Can you work these out from the model? Positions are in its coordinate system, mm. A direction names the side the tool comes from. Give positions to 0.01 mm unless a question says otherwise; leave off trailing zeros. Order: outer loops, then holes, each group sorted by start corner. A loop starts at its lowest first (then second) coordinate and runs counter-clockwise, first axis right, second up. Notation, with made-up numbers: M 15.5,-22.5 L 20.5,-22.5 A19 cw 20.5,9.5 Z; hole C 62,-14 d11. An arc over 180 degrees is marked long. One line per question, with ' | ' between items. Start each with the question number.
1) I'm going to push flat-ended pins straight in: pin 1 Ø10 at (y, z) = (-773, 4.5) entering from +X; pin 2 Ø5 at (x, z) = (-20.5, 11) entering from -Y; pin 3 Ø5 at (y, z) = (-780, 2) entering from -X. Where does each tip first touch, or does it pass through?
2) If we section it at C-C, the plane y = -778: Please give me the cut outline in (x, z) (3 decimals).
3) If we section it at B-B, the plane x = -28: Please give me the cut outline in (y, z) (3 decimals), plus the area to 3 significant figures.
4) If we section it at A-A, the plane z = 0: Please give me the cut outline in (x, y).
5) For faces 4 (the flat face through (-16, -775, -9.525)), 5 (the cylindrical face through (-7.9, -759.1, -12.1)), which set-ups out of +Z, -Z, +X, -X, +Y, -Y let a thin tool reach every point of the face, with its end or its side?
6) If we section it at D-D, the plane y = -766.5: Please give me the cut outline in (x, z) (3 decimals).
7) Please list where these lines run through material, in increasing order: line 1 along Z through (x, y) = (-9, -783) (3 decimals); line 2 along X through (y, z) = (-762.5, -2.5); line 3 along Y through (x, z) = (-27.5, -10.5). Write a range as [from, to].
8) Thinking about a two-plate mould opening in Y: for faces 1 (the flat face through (-3, -759.052, 0)), 2 (the cylindrical face through (-23.005, -779.083, 12.101)), 3 (the flat face through (-34.362, -776, 12)), which applies, +Y half, -Y half, draft (parallel to the pull), parting line (faces both ways), or undercut?
```python
from build123d import *

# Parameters (mm, degrees)
BOSS_EXTRUDE1_DEPTH = 33.02
CUT_EXTRUDE1_REACH  = 794.952
SKETCH2_R           = 3.175
SKETCH3_R           = 3.96875
CUT_EXTRUDE2_DEPTH  = 794.354962335
FILLET1_R           = 3.175


with BuildPart() as part:
    # Sketch1 → Boss-Extrude1 (new body)
    with BuildSketch(Plane(origin=(0, -759.052062329, 0), x_dir=(-1, 0, 0), z_dir=(0, -1, 0))):
        Polygon((0, 14.605), (0, -14.605), (34.361609966, -14.605), (34.361609966, -9.525), (5.08, -9.525), (5.08, 9.525), (34.361609966, 9.525), (34.361609966, 14.605), align=None)
    extrude(amount=BOSS_EXTRUDE1_DEPTH)

    # Sketch2 → Cut-Extrude1 (cut, up to next)
    with BuildSketch(Plane(origin=(0, 0, 0), x_dir=(0, 0, -1), z_dir=(1, 0, 0)), mode=Mode.PRIVATE) as cut_extrude1_sk1:
        with Locations(Location((0, -784.452062329, 0), (0, 0, 90))):
            Circle(SKETCH2_R)
    cut_extrude1_tool1 = extrude(cut_extrude1_sk1.sketch, amount=-CUT_EXTRUDE1_REACH, mode=Mode.PRIVATE) & part.part
    # Sketch2 → Cut-Extrude1 (cut, up to next)
    with BuildSketch(Plane(origin=(0, 0, 0), x_dir=(0, 0, -1), z_dir=(1, 0, 0)), mode=Mode.PRIVATE) as cut_extrude1_sk2:
        with Locations(Location((0, -766.672062329, 0), (0, 0, 90))):
            Circle(SKETCH2_R)
    cut_extrude1_tool2 = extrude(cut_extrude1_sk2.sketch, amount=-CUT_EXTRUDE1_REACH, mode=Mode.PRIVATE) & part.part
    add(cut_extrude1_tool1.solids().sort_by_distance((0, -784.452062, 0))[0], mode=Mode.SUBTRACT)
    add(cut_extrude1_tool2.solids().sort_by_distance((0, -766.672062, 0))[0], mode=Mode.SUBTRACT)

    # Sketch3 → Cut-Extrude2 (cut, through all)
    with BuildSketch(Plane.XY.offset(14.605)):
        with Locations((-24.836609966, -775.562062329)):
            Circle(SKETCH3_R)
        Polygon((-7.9375, -759.052062329), (-34.361609966, -769.212062329), (-34.361609966, -759.052062329), align=None)
        Polygon((-34.361609966, -792.072062329), (-34.361609966, -781.912062329), (-7.9375, -792.072062329), align=None)
    extrude(amount=-CUT_EXTRUDE2_DEPTH, mode=Mode.SUBTRACT)

    # Fillet1
    fillet1_edges = [part.edges().sort_by_distance(p)[0] for p in [
        (-7.9375, -759.052062329, 12.065),
        (-7.9375, -792.072062329, 12.065),
        (-34.361609966, -781.912062329, 12.065),
        (-7.9375, -792.072062329, -12.065),
        (-34.361609966, -781.912062329, -12.065),
        (-34.361609966, -769.212062329, 12.065),
        (-7.9375, -759.052062329, -12.065),
        (-34.361609966, -769.212062329, -12.065),
    ]]
    fillet(fillet1_edges, radius=FILLET1_R)


solid = part.part
```
Results found:
1) pin 1: stops at x = 0 | pin 2: stops at y = -788.2 | pin 3: stops at x = -5.08
2) outline: M -34.362,-14.605 L -27.968,-14.605 L -27.968,-9.525 L -34.362,-9.525 Z; M -34.362,9.525 L -27.968,9.525 L -27.968,14.605 L -34.362,14.605 Z; M -21.705,-14.605 L 0,-14.605 L 0,14.605 L -21.705,14.605 L -21.705,9.525 L -5.08,9.525 L -5.08,-9.525 L -21.705,-9.525 Z
3) outline: M -784.358,-14.605 L -777.959,-14.605 L -777.959,-9.525 L -784.358,-9.525 Z; M -784.358,9.525 L -777.959,9.525 L -777.959,14.605 L -784.358,14.605 Z; M -773.165,-14.605 L -766.766,-14.605 L -766.766,-9.525 L -773.165,-9.525 Z; M -773.165,9.525 L -766.766,9.525 L -766.766,14.605 L -773.165,14.605 Z | area: 130 mm²
4) outline: M -5.08,-792.07 L 0,-792.07 L 0,-787.63 L -5.08,-787.63 Z; M -5.08,-781.28 L 0,-781.28 L 0,-769.85 L -5.08,-769.85 Z; M -5.08,-763.5 L 0,-763.5 L 0,-759.05 L -5.08,-759.05 Z
5) face 4: -X, +Y, -Y | face 5: +Z, -Z, -X, +Y
6) outline: M -27.308,-14.605 L 0,-14.605 L 0,-3.17 L -5.08,-3.17 L -5.08,-9.525 L -27.308,-9.525 Z; M -27.308,9.525 L -5.08,9.525 L -5.08,3.17 L 0,3.17 L 0,14.605 L -27.308,14.605 Z
7) line 1: z = [-14.605, -9.525], [9.525, 14.605] | line 2: x = [-5.08, 0] | line 3: y = [-784.55, -778.5], [-772.62, -766.57]
8) face 1: +Y half | face 2: undercut | face 3: draft
